```python
from build123d import *

# Parameters (mm, degrees)
F0_W     = 150
F0_H     = 100
F1_DEPTH = 20
F2_R     = 17.5
F3_DEPTH = 15
F5_D     = 10


with BuildPart() as f1:
    # F0 (on Top) → F1 (new body)
    with BuildSketch(Plane.XY):
        Rectangle(F0_W, F0_H)
    extrude(amount=F1_DEPTH)

    # F2 (on face) → F3 (join)
    with BuildSketch(Plane.XY.offset(20)):
        Circle(F2_R)
    extrude(amount=F3_DEPTH)

    # F5 (through all)
    with Locations(Plane.XY.offset(20)):
        with Locations((-65, 40)):
            Hole(F5_D / 2)


solid = f1.part
```
Verification items for the finished model (mm, model axes). Give positions to 0.01 mm unless a question says otherwise; leave off trailing zeros. Order: outer loops, then holes, each group sorted by start corner. A loop starts at its lowest first (then second) coordinate and runs counter-clockwise, first axis right, second up. Notation, with made-up numbers: M 71,84.5 L 88,84.5 A13 ccw 88,98.5 Z; hole C 13.25,1.5 d4. An arc over 180 degrees is marked long. Answer in a Markdown table with one row per item. Add a question column.
Item 1: Mould release check, pull along X, two halves, no side actions. Record for faces 1 (the flat face through (-1, 50, 10)), 2 (the cylindrical face through (-64.349, 44.957, 9.86)), 3 (the cylindrical face through (-13.887, -10.648, 27.395)), 4 (the flat face through (75, -1, 10)): released by +X, released by -X, zero draft, split by the parting line, or undercut.
Item 2: Section check C-C, the plane x = 0. Enter the section's corners in (y, z).
Item 3: Section check D-D, the plane y = 0. Enter the section's corners in (x, z), and give its area (4 significant figures).
Item 4: Scan lines: probe 1 along Y at (x, z) = (-65, 15); probe 2 along Z at (x, y) = (10.5, -23.5); probe 3 along Y at (x, z) = (-0.5, 27). Record each from-to range of solid material in increasing order. Write a range as from..to.
Item 5: Section check A-A, the plane y = 40. Enter the section's corners in (x, z).
Item 6: Section check B-B, the plane x = -65. Enter the section's corners in (y, z), and give its area (3 significant figures).
Filled sheet:
| question | item | result |
|---|---|---|
| 1 | face 1 | zero draft |
| 1 | face 2 | undercut |
| 1 | face 3 | split by the parting line |
| 1 | face 4 | released by +X |
| 2 | outline | M -50,0 L 50,0 L 50,20 L 17.5,20 L 17.5,35 L -17.5,35 L -17.5,20 L -50,20 Z |
| 3 | outline | M -75,0 L 75,0 L 75,20 L 17.5,20 L 17.5,35 L -17.5,35 L -17.5,20 L -75,20 Z |
| 3 | area | 3,525 mm^2 |
| 4 | probe 1 | y = -50..35, 45..50 |
| 4 | probe 2 | z = 0..20 |
| 4 | probe 3 | y = -17.49..17.49 |
| 5 | outline | M -75,0 L -70,0 L -70,20 L -75,20 Z; M -60,0 L 75,0 L 75,20 L -60,20 Z |
| 6 | outline | M -50,0 L 35,0 L 35,20 L -50,20 Z; M 45,0 L 50,0 L 50,20 L 45,20 Z |
| 6 | area | 1,800 mm^2 |
